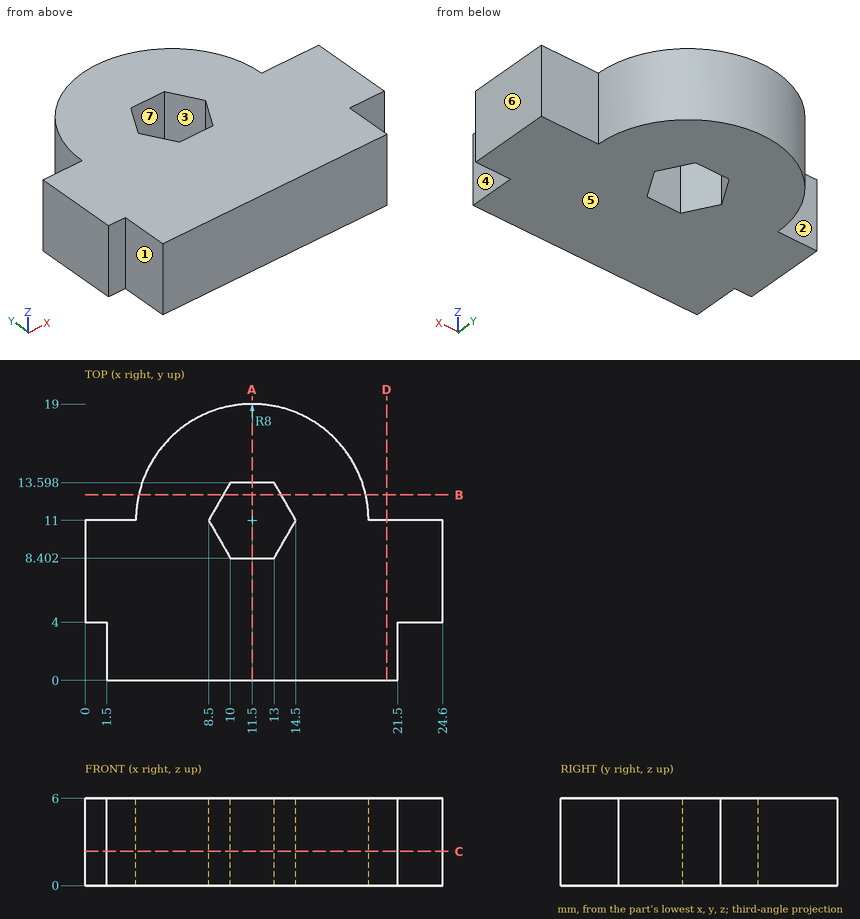
Geometry: see drawing. Coordinates: mm, zero at the bounding-box minimum. A direction names the side the tool comes from. Give positions to 0.01 mm unless a question says otherwise; leave off trailing zeros. Order: outer loops, then holes, each group sorted by start corner. A loop starts at its lowest first (then second) coordinate and runs counter-clockwise, first axis right, second up. Notation, with made-up numbers: (-23, -16.75) -> (19, -16.75) arc R18 cw to (19, 8.25) -> close; hole circle Ø5 at (76, -14). An arc over 180 degrees is marked (long way). Write item = value, one per line.
Q1. Pin query (flat end, axial travel): pin 1 (1.2 mm diameter, centred on y = 2, z = 3, fed in from +X); pin 2 (3.5 mm diameter, centred on x = 22.5, z = 3, fed in from -Y); pin 3 (3 mm diameter, centred on x = 1, z = 3, fed in from +Y); pin 4 (3 mm diameter, centred on x = 9, z = 4.5, fed in from +Y). Return the tip coordinate at first contact, or that it passes through.
Data:
pin_1 = 21.5
pin_2 = 0
pin_3 = 11
pin_4 = 18.94
Q2. Cut plane D-D, the plane x = 20.75. Output: boundary loops of the cut face in (y, z), and give its area (3 significant figures).
Data:
outline = (0, 0) -> (11, 0) -> (11, 6) -> (0, 6) -> close
area = 66.0 mm^2
Q3. Material intervals for line 1 (X direction, y = 2, z = 2.5); line 2 (X direction, y = 12.75, z = 4.7); line 3 (X direction, y = 13, z = 1.3) (1 decimal), sorted ascending. Write a range as from..to.
Data:
line_1 = 1.5..21.5
line_2 = 3.69..9.51, 13.49..19.31
line_3 = 3.8..9.7, 13.3..19.2
Q4. Pull-direction query (X, two-part tool) for the marked faces 5, 6 and 7; classes: released by +X, released by -X, zero draft, split by the parting line, or undercut.
Data:
face_5 = zero draft
face_6 = released by +X
face_7 = undercut
Q5. Cut plane A-A, the plane x = 11.5. Output: boundary loops of the cut face in (y, z).
Data:
outline = (0, 0) -> (8.4, 0) -> (8.4, 6) -> (0, 6) -> close; (13.6, 0) -> (19, 0) -> (19, 6) -> (13.6, 6) -> close
Q6. Set-up query: the marked faces 1, 2, 3 and 4. Return all of +Z, -Z, +X, -X, +Y, -Y with unobstructed straight access to the full face (end or side cutting, diameter ignored); none if empty.
Data:
face_1 = +Z, -Z, -X, -Y
face_2 = +Z, -Z, -X, +Y
face_3 = +Z, -Z
face_4 = +Z, -Z, +X, -Y
Q7. Cut plane B-B, the plane y = 12.75. Output: boundary loops of the cut face in (x, z), and give its area (3 significant figures).
Data:
outline = (3.69, 0) -> (9.51, 0) -> (9.51, 6) -> (3.69, 6) -> close; (13.49, 0) -> (19.31, 0) -> (19.31, 6) -> (13.49, 6) -> close
area = 69.8 mm^2
Q8. Cut plane C-C, the plane z = 2.35. Output: boundary loops of the cut face in (x, y).
Data:
outline = (0, 4) -> (1.5, 4) -> (1.5, 0) -> (21.5, 0) -> (21.5, 4) -> (24.6, 4) -> (24.6, 11) -> (19.5, 11) arc R8 ccw to (3.5, 11) -> (0, 11) -> close; hole (8.5, 11) -> (10, 8.4) -> (13, 8.4) -> (14.5, 11) -> (13, 13.6) -> (10, 13.6) -> close
